from build123d import *

# Parameters (mm, degrees)
SKETCH1_R           = 1.4732
BOSS_EXTRUDE1_DEPTH = 3.2004
SKETCH2_W           = 1.27
SKETCH2_H           = 0.508
CUT_EXTRUDE1_DEPTH  = 3.2004
SKETCH3_R           = 2.159
CUT_EXTRUDE2_DEPTH  = 3.2004


with BuildPart() as part:
    # Sketch1 → Boss-Extrude1 (new body)
    with BuildSketch(Plane.XY):
        with BuildLine():
            Line((1.58185229, 18.90776), (84.13185229, 12.0015))
            ThreePointArc((84.13185229, 12.0015), (95.171215867, 0), (84.13185229, -12.0015))
            Line((84.13185229, -12.0015), (1.58185229, -18.90776))
            ThreePointArc((1.58185229, -18.90776), (-18.973814716, 0), (1.58185229, 18.90776))
        make_face()
        Circle(SKETCH1_R, mode=Mode.SUBTRACT)
    extrude(amount=BOSS_EXTRUDE1_DEPTH)

    # Sketch2 → Cut-Extrude1 (cut)
    with BuildSketch(Plane.XY.offset(3.2004)):
        Polygon((-4.582879775, -14.447974492), (-4.409133542, -13.970610641), (-5.602543171, -13.536245059), (-5.776289403, -14.01360891), align=None)
        with Locations((0, -14.890092213)):
            Rectangle(SKETCH2_W, SKETCH2_H)
    extrude(amount=-CUT_EXTRUDE1_DEPTH, mode=Mode.SUBTRACT)

    # Sketch3 → Cut-Extrude2 (cut)
    with BuildSketch(Plane.XY.offset(3.2004)):
        with Locations((0, 8.89)):
            Circle(SKETCH3_R)
        with Locations((7.69896584, -4.445)):
            Circle(SKETCH3_R)
        with Locations((-7.69896584, -4.445)):
            Circle(SKETCH3_R)
    extrude(amount=-CUT_EXTRUDE2_DEPTH, mode=Mode.SUBTRACT)


solid = part.part
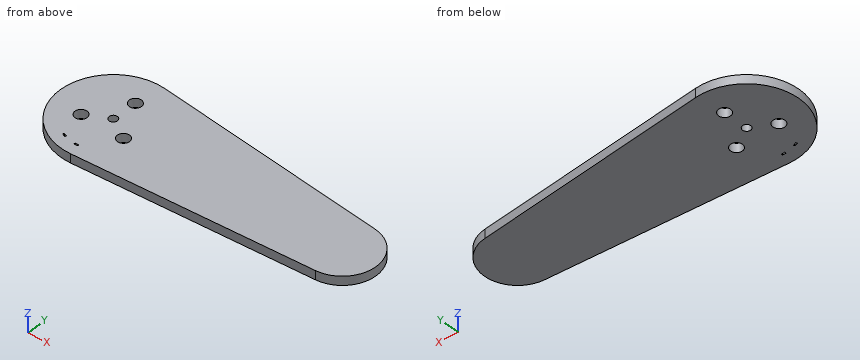
Input: part model. Units: mm. Frame: model coordinates. Round coordinates to 2 decimals unless told otherwise and drop trailing zeros. Loops run counter-clockwise (first coordinate to the right, second up) from the corner with the lowest first, then second, coordinate; pieces in that order, holes last. Notation, with made-up numbers: M 53.5,-38 L 101.5,-38 A12 ccw 101.5,-22 Z; hole C -32.5,13.5 d4. An arc over 180 degrees is marked long. Answer as CSV lines item,"result". Start each with the question number.
(1) Section A-A, the plane y = 0. Output: boundary loops of the cut face in (x, z), plus the area to 3 significant figures.
(2) Section B-B, the plane x = 39.5. Output: boundary loops of the cut face in (y, z).
(3) First-contact query: pin 1 (3.5 mm diameter, centred on x = 0, y = 8.89, fed in from -Z); pin 2 (1 mm diameter, centred on y = 1.5, z = 1.5, fed in from -X); pin 3 (1 mm diameter, centred on y = -3, z = 2.5, fed in from -X). Flat tips, straight axial feed; report the tip coordinate or a pass-through.
(4) Section D-D, the plane x = 74.5. Output: boundary loops of the cut face in (y, z), plus the area to 3 significant figures.
(5) Section C-C, the plane y = 8.89. Output: boundary loops of the cut face in (x, z).
(6) Line query: line 1 (Y direction, x = 0, z = 1.75); line 2 (X direction, y = -5, z = 0.2); line 3 (Y direction, x = 86, z = 0.6). Output: solid intervals per line, ascending. Write a range as [from, to].
Values found:
1,outline,"M -18.97,0 L -1.47,0 L -1.47,3.2 L -18.97,3.2 Z; M 1.47,0 L 95.17,0 L 95.17,3.2 L 1.47,3.2 Z"
1,area,"356 mm²"
2,outline,"M -15.74,0 L 15.74,0 L 15.74,3.2 L -15.74,3.2 Z"
3,pin 1,"passes through"
3,pin 2,"stops at x = -18.95"
3,pin 3,"stops at x = -18.81"
4,outline,"M -12.81,0 L 12.81,0 L 12.81,3.2 L -12.81,3.2 Z"
4,area,"82.0 mm²"
5,outline,"M -16.76,0 L -2.16,0 L -2.16,3.2 L -16.76,3.2 Z; M 2.16,0 L 91.25,0 L 91.25,3.2 L 2.16,3.2 Z"
6,line 1,"y = [-18.97, -15.14], [-14.64, -1.47], [1.47, 6.73], [11.05, 18.97]"
6,line 2,"x = [-18.3, -9.79], [-5.61, 5.61], [9.79, 94.08]"
6,line 3,"y = [-11.7, 11.7]"
